```python
from build123d import *

# Parameters (mm, degrees)
EXTRUDE_1_DEPTH            = 4
SKETCH_4_W                 = 1.5
SKETCH_4_H                 = 8
SKETCH_4_W_2               = 8
SKETCH_4_H_2               = 1.5
EXTRUDE_2_DEPTH            = 1
MIRROR_2_COPY_1_DEPTH      = 4
MIRROR_2_COPY_3_SKETCH_W   = 1.5
MIRROR_2_COPY_3_SKETCH_H   = 8
MIRROR_2_COPY_3_SKETCH_W_2 = 8
MIRROR_2_COPY_3_SKETCH_H_2 = 1.5
MIRROR_2_COPY_3_DEPTH      = 1


with BuildPart() as part:
    # Эскиз1 → Бобышка-Вытянуть1 (new body)
    with BuildSketch(Plane.XY):
        with BuildLine():
            Line((0, 0), (0, 38))
            Line((0, 38), (4, 38))
            ThreePointArc((4, 38), (28.04163056, 28.04163056), (38, 4))
            Line((38, 4), (38, 0))
            Line((38, 0), (0, 0))
        make_face()
    extrude_1 = extrude(amount=EXTRUDE_1_DEPTH)

    # Эскиз3 → Зенковка для винта с полупотайной головкой M81 (revolve, cut)
    with BuildSketch(Plane(origin=(20, 20, 4), x_dir=(0, -1, 0), z_dir=(1, 0, 0))):
        Polygon((0, 0), (0, 11.953872786), (4.5, 9.25), (4.5, 3.5), (8, 0), align=None)
    hole_wizard_m81 = revolve(axis=Axis((20, 20, 10.35), (0, 0, -1)), mode=Mode.SUBTRACT)

    # Эскиз4 → Бобышка-Вытянуть2 (add)
    with BuildSketch(Plane(origin=(0, 0, 0), x_dir=(-1, 0, 0), z_dir=(0, 0, -1))):
        with Locations((-2.25, 20)):
            Rectangle(SKETCH_4_W, SKETCH_4_H)
        with Locations((-20, 2.25)):
            Rectangle(SKETCH_4_W_2, SKETCH_4_H_2)
    extrude_2 = extrude(amount=EXTRUDE_2_DEPTH)

    # Зеркальное отражение1: Бобышка-Вытянуть1, Зенковка для винта с полупотайной головкой M81, Бобышка-Вытянуть2 across plane
    add(extrude_1.mirror(Plane(origin=(0, 0, 0), x_dir=(0, 0.707106781, 0.707106781), z_dir=(0, -0.707106781, 0.707106781))))
    add(hole_wizard_m81.mirror(Plane(origin=(0, 0, 0), x_dir=(0, 0.707106781, 0.707106781), z_dir=(0, -0.707106781, 0.707106781))), mode=Mode.SUBTRACT)
    add(extrude_2.mirror(Plane(origin=(0, 0, 0), x_dir=(0, 0.707106781, 0.707106781), z_dir=(0, -0.707106781, 0.707106781))))

    # Зеркальное отражение2: Бобышка-Вытянуть1, Зенковка для винта с полупотайной головкой M81, Бобышка-Вытянуть2 across plane
    add(extrude_1.mirror(Plane(origin=(0, 0, 0), x_dir=(0.707106781, 0, 0.707106781), z_dir=(-0.707106781, 0, 0.707106781))))
    add(hole_wizard_m81.mirror(Plane(origin=(0, 0, 0), x_dir=(0.707106781, 0, 0.707106781), z_dir=(-0.707106781, 0, 0.707106781))), mode=Mode.SUBTRACT)
    add(extrude_2.mirror(Plane(origin=(0, 0, 0), x_dir=(0.707106781, 0, 0.707106781), z_dir=(-0.707106781, 0, 0.707106781))))

    # Зеркальное отражение2 copy 1 sketch → Зеркальное отражение2 copy 1 (add)
    with BuildSketch(Plane.ZX):
        with BuildLine():
            Line((0, 0), (0, 38))
            Line((0, 38), (4, 38))
            ThreePointArc((4, 38), (28.04163056, 28.04163056), (38, 4))
            Line((38, 4), (38, 0))
            Line((38, 0), (0, 0))
        make_face()
    extrude(amount=MIRROR_2_COPY_1_DEPTH)

    # Зеркальное отражение2 copy 2 sketch → Зеркальное отражение2 copy 2 (revolve, cut)
    with BuildSketch(Plane(origin=(20, 4, 20), x_dir=(-1, 0, 0), z_dir=(0, 0, 1))):
        Polygon((0, 0), (0, 11.953872786), (4.5, 9.25), (4.5, 3.5), (8, 0), align=None)
    revolve(axis=Axis((20, 10.35, 20), (0, -1, 0)), mode=Mode.SUBTRACT)

    # Зеркальное отражение2 copy 3 sketch → Зеркальное отражение2 copy 3 (add)
    with BuildSketch(Plane(origin=(0, 0, 0), x_dir=(0, 0, -1), z_dir=(0, -1, 0))):
        with Locations((-2.25, 20)):
            Rectangle(MIRROR_2_COPY_3_SKETCH_W, MIRROR_2_COPY_3_SKETCH_H)
        with Locations((-20, 2.25)):
            Rectangle(MIRROR_2_COPY_3_SKETCH_W_2, MIRROR_2_COPY_3_SKETCH_H_2)
    extrude(amount=MIRROR_2_COPY_3_DEPTH)


solid = part.part
```
Geometry: final body of the model. Coordinates: model frame, mm. A direction names the side the tool comes from. Round coordinates to 2 decimals unless told otherwise and drop trailing zeros. Order: outer loops, then holes, each group sorted by start corner. A loop starts at its lowest first (then second) coordinate and runs counter-clockwise, first axis right, second up. Notation, with made-up numbers: M -11,61 L 8,61 A15 cw 8,67 Z; hole C 70,62.5 d3. An arc over 180 degrees is marked long. Use one line per item in the form item = value. Start each with the question number.
Q1. Cut plane D-D (x = 31). Return loops of the section in (y, z).
Q2. Mould query, pull axis Y, two halves, no side actions, for faces 1 (the face through (-1, 2, 20)), 2 (the face through (16.96, 23.32, 0.25)), 3 (the face through (2, 38, 2)). Classes: +Y half, -Y half, draft (parallel to the pull), parting line (faces both ways), or undercut.
Q3. Pin query (flat end, axial travel): pin 1 Ø1.5 at (x, y) = (9.5, 13.5) entering from +Z; pin 2 Ø0.5 at (x, y) = (-0.5, 20) entering from -Z; pin 3 Ø10 at (y, z) = (14.5, 23.5) entering from +X. Return the tip coordinate at first contact, or that it passes through.
Q4. Material intervals for line 1 (X direction, y = 36, z = 5), sorted ascending. Write a range as [from, to].
Q5. Cut plane A-A (z = 20). Return loops of the section in (x, y).
Q6. Cut plane C-C (z = 33.5). Return loops of the section in (x, y), and give its area (3 significant figures).
Q7. Access query for faces 4 (the face through (2, -1, 20)), 5 (the face through (4, 14, 14)). Directions: +Z, -Z, +X, -X, +Y, -Y. A direction counts if a zero-diameter tool reaches every point of the face in a straight line with its end or side. Return the directions, or none.
Geometry results:
q1.outline = M 0,0 L 24.66,0 L 24.66,4 L 4,4 L 4,24.66 L 0,24.66 Z
q2.face_1 = draft
q2.face_2 = undercut
q2.face_3 = +Y half
q3.pin_1 = 4
q3.pin_2 = 1.5
q3.pin_3 = 4
q4.line_1 = [0, 4]
q5.outline = M -1,1.5 L 0,1.5 L 0,0 L 1.5,0 L 1.5,-1 L 3,-1 L 3,0 L 15.5,0 L 15.5,0.5 L 12,4 L 4,4 L 4,12 L 0.5,15.5 L 0,15.5 L 0,3 L -1,3 Z; M 0,24.5 L 0.5,24.5 L 4,28 L 4,34 L 0,34 Z; M 24.5,0 L 34,0 L 34,4 L 28,4 L 24.5,0.5 Z
q6.outline = M 0,0 L 20.9,0 L 20.9,4 L 4,4 L 4,20.9 L 0,20.9 Z
q6.area = 151 mm^2
q7.face_4 = +Z, -Z, +X, -X, -Y
q7.face_5 = +Z, +X, +Y
